```python
from build123d import *

# Parameters (mm, degrees)
BOSS_EXTRUDE1_DEPTH = 25
SKETCH2_R           = 3
CUT_EXTRUDE1_DEPTH  = 108.652217813
SKETCH3_R           = 2.5
CUT_EXTRUDE2_DEPTH  = 20
FILLET2_R           = 13


with BuildPart() as part:
    # Sketch1 → Boss-Extrude1 (new body)
    with BuildSketch(Plane.XY):
        Polygon((0, 50), (10, 50), (10, 10), (82, 10), (82, 50), (92, 50), (92, 0), (0, 0), align=None)
    extrude(amount=BOSS_EXTRUDE1_DEPTH)

    # Sketch2 → Cut-Extrude1 (cut, through all)
    with BuildSketch(Plane(origin=(92, 0, 0), x_dir=(0, 0, -1), z_dir=(1, 0, 0))):
        with Locations((-12.5, 40)):
            Circle(SKETCH2_R)
    extrude(amount=-CUT_EXTRUDE1_DEPTH, mode=Mode.SUBTRACT)

    # Sketch3 → Cut-Extrude2 (cut)
    with BuildSketch(Plane(origin=(0, 10, 0), x_dir=(1, 0, 0), z_dir=(0, 1, 0))):
        with Locations(Location((20, -12.5, 0), (0, 0, 270))):
            Circle(SKETCH3_R)
        with Locations(Location((72, -12.5, 0), (0, 0, 270))):
            Circle(SKETCH3_R)
    extrude(amount=-CUT_EXTRUDE2_DEPTH, mode=Mode.SUBTRACT)

    # Fillet2
    # the kernel refuses this fillet: 13 mm, written as the material it takes off along each edge
    with BuildSketch(Plane(origin=(49.5, 50, 0), x_dir=(0, -1, 0), z_dir=(1, 0, 0)), Plane(origin=(-32.5, 50, 25), x_dir=(0, 0, -1), z_dir=(1, 0, 0))) as fillet2_piece_1:
        with BuildLine():
            CenterArc((FILLET2_R, -FILLET2_R), FILLET2_R, 90, 90)
            Line((0, -FILLET2_R), (0, 0))
            Line((0, 0), (FILLET2_R, 0))
        make_face()
    extrude(amount=75, mode=Mode.SUBTRACT)
    with BuildSketch(Plane(origin=(49.5, 50, 25), x_dir=(0, -1, 0), z_dir=(1, 0, 0)), Plane(origin=(-32.5, 50, 0), x_dir=(0, 0, 1), z_dir=(1, 0, 0))) as fillet2_piece_2:
        with BuildLine():
            CenterArc((FILLET2_R, FILLET2_R), FILLET2_R, 180, 90)
            Line((0, FILLET2_R), (0, 0))
            Line((0, 0), (FILLET2_R, 0))
        make_face()
    extrude(amount=75, mode=Mode.SUBTRACT)


solid = part.part
```
Model file for the job. Use its own axes, mm. A direction names the side the tool comes from. Give positions to 0.01 mm unless a question says otherwise; leave off trailing zeros. Loops run counter-clockwise (first coordinate to the right, second up) from the corner with the lowest first, then second, coordinate; pieces in that order, holes last. Notation, with made-up numbers: (-38.75, 55) -> (-17.75, 55) arc R12 cw to (-17.75, 59) -> close; hole circle Ø2 at (50.5, 80.25). An arc over 180 degrees is marked (long way). Use CSV: the item, a comma, the result in double quotes. Start each with the question number.
1) Flat gauge pin, fed straight in: pin 1 Ø8 at (x, z) = (20, 12.5) entering from +Y. Where does the tip first touch, or does it go through?
2) Wall check: line 1 (X direction, y = 5.25, z = 12.5); line 2 (X direction, y = 12, z = 24); line 3 (X direction, y = 3, z = 14.75). Give the ranges that are in metal, low to high.
3) Slice it at B-B on y = 22. Give the cut face in (x, z), plus the area to 3 significant figures.
4) Slice it at A-A on x = 20. Give the cut face in (y, z), plus the area to 3 significant figures.
5) Mould opens along Y. For faces 3 (the flat face through (10, 30, 12)), 4 (the cylindrical face through (5.07, 42.03, 14.71)), 5 (the cylindrical face through (4.93, 46.114, 21.27)), 6 (the cylindrical face through (87.07, 42.03, 14.71)) say: released by +Y, released by -Y, zero draft, split by the parting line, or undercut.
6) Tool access for faces 1 (the cylindrical face through (4.93, 45.913, 3.536)), 2 (the flat face through (45, 10, 12)): list every direction of +Z, -Z, +X, -X, +Y, -Y with a clear straight run to the whole face (end or side of a thin tool).
7) Slice it at D-D on z = 21. Give the cut face in (x, y).
8) Slice it at C-C on y = 40. Give the cut face in (x, z).
Computed values:
1,pin 1,"stops at y = 10"
2,line 1,"x = 0 to 17.5, 22.5 to 69.5, 74.5 to 92"
2,line 2,"x = 0 to 10, 82 to 92"
2,line 3,"x = 0 to 18.91, 21.09 to 70.91, 73.09 to 92"
3,outline,"(0, 0) -> (10, 0) -> (10, 25) -> (0, 25) -> close; (82, 0) -> (92, 0) -> (92, 25) -> (82, 25) -> close"
3,area,"500 mm^2"
4,outline,"(0, 0) -> (10, 0) -> (10, 10) -> (0, 10) -> close; (0, 15) -> (10, 15) -> (10, 25) -> (0, 25) -> close"
4,area,"200 mm^2"
5,face 3,"zero draft"
5,face 4,"undercut"
5,face 5,"released by +Y"
5,face 6,"undercut"
6,face 1,"-Z, +X, -X, +Y"
6,face 2,"+Z, -Z, +Y"
7,outline,"(0, 0) -> (92, 0) -> (92, 46.38) -> (82, 46.38) -> (82, 10) -> (10, 10) -> (10, 46.38) -> (0, 46.38) -> close"
8,outline,"(0, 0.35) -> (10, 0.35) -> (10, 9.5) -> (0, 9.5) -> close; (0, 15.5) -> (10, 15.5) -> (10, 24.65) -> (0, 24.65) -> close; (82, 0.35) -> (92, 0.35) -> (92, 9.5) -> (82, 9.5) -> close; (82, 15.5) -> (92, 15.5) -> (92, 24.65) -> (82, 24.65) -> close"
